CAD build for the part. Positions are in the model's coordinates, mm. A direction names the side the tool comes from. Give positions to 0.01 mm unless a question says otherwise; leave off trailing zeros. Order: outer loops, then holes, each group sorted by start corner. A loop starts at its lowest first (then second) coordinate and runs counter-clockwise, first axis right, second up. Notation, with made-up numbers: (25.5, 42) -> (83.5, 42) arc R23 cw to (83.5, 57) -> close; hole circle Ø11 at (3, 54.5). An arc over 180 degrees is marked (long way). Answer as CSV lines item,"result".
Autodesk Inventor part; units mm, degrees
sketch "Skizze1" plane through (0, 0, 0) normal (0, 1, 0) x (-1, 0, 0)
  line L0 (75, 67.5) -> (-75, 67.5)
  line L1 (-75, 67.5) -> (-75, -67.5)
  line L2 (-75, -67.5) -> (75, -67.5)
  line L3 (75, -67.5) -> (75, 67.5)
  line L4 (75, 67.5) -> (-75, -67.5) construction
  line L5 (-75, 67.5) -> (75, -67.5) construction
  point P0 (0, 0)
  dimension "d0" = 150
  dimension "d1" = 135
extrude "Extrusion1" add sketch "Skizze1" along normal mid plane 3
sketch "Skizze2" plane through (0, 1.5, 0) normal (0, 1, 0) x (1, 0, 0)
  line L0 (-75, 67.5) -> (-75, -67.5)
  line L1 (75, -67.5) -> (75, 67.5)
  line L2 (-75, -67.5) -> (75, -67.5)
  line L3 (75, -67.5) -> (75, -66)
  line L4 (75, -66) -> (-75, -66)
  line L5 (-75, -66) -> (-75, -67.5)
  point P0 (0, 0)
  dimension "d4" = 135
  dimension "d5" = 1.5
extrude "Extrusion2" add sketch "Skizze2" along normal blind 15
sketch "Skizze3" plane through (0, 0, 0) normal (1, 0, 0) x (0, 1, 0)
  line L0 (1.5, -67.5) -> (1.5, 66)
  line L1 (1.5, -67.5) -> (-1.5, -67.5)
  line L2 (-1.5, -67.5) -> (-1.5, -77.5)
  line L3 (-1.5, -77.5) -> (1.5, -77.5)
  line L4 (1.5, -77.5) -> (1.5, -67.5)
  line L5 (2, -78.5) -> (11.5, -78.5)
  line L6 (1.5, -77.5) -> (1.5, -78)
  line L7 (-1.5, -77.5) -> (-1.5, -79.5)
  arc A0 (1.5, -78) -> (2, -78.5) centre (2, -78) ccw
  line L8 (12, -78.5) -> (12, -80)
  line L9 (12, -80) -> (-1, -80)
  arc A1 (-1.5, -79.5) -> (-1, -80) centre (-1, -79.5) ccw
  line L10 (12, -78) -> (12, -78)
  arc A2 (11.5, -78.5) -> (12, -78) centre (11.5, -78) ccw
  line L11 (12, -78.5) -> (12, -78)
  point P0 (0, 0)
  dimension "d8" = 10
  dimension "d16" = 1.5
  dimension "d17" = 0.5
  dimension "d19" = 10
  dimension "d20" = 0.5
extrude "Extrusion3" add sketch "Skizze3" along normal mid plane 150
sketch "Skizze5" plane through (0, 0, 0) normal (0, 0, 1) x (1, 0, 0)
  line L0 (75, 16.5) -> (75, -1.5)
  line L1 (75, -1.5) -> (87, -1.5)
  line L2 (87.5, -1) -> (87.5, 12)
  line L3 (85.5, 12) -> (85.5, 12)
  line L4 (86, 11.5) -> (86, 2)
  arc A0 (86, 11.5) -> (85.5, 12) centre (85.5, 11.5) ccw
  line L5 (85.5, 12) -> (87.5, 12)
  line L6 (75, 1.5) -> (85.5, 1.5)
  line L7 (75, -1.5) -> (-75, -1.5)
  line L8 (75, -1.5) -> (75, 1.5)
  arc A1 (85.5, 1.5) -> (86, 2) centre (85.5, 2) ccw
  arc A2 (87, -1.5) -> (87.5, -1) centre (87, -1) ccw
  line L9 (-75, -1.5) -> (-75, 16.5)
  line L10 (-75, -1.5) -> (-87, -1.5)
  line L11 (-87.5, -1) -> (-87.5, 12)
  line L12 (-85.5, 12) -> (-85.5, 12)
  line L13 (-86, 11.5) -> (-86, 2)
  line L14 (-85.5, 1.5) -> (-75, 1.5)
  line L15 (-75, 1.5) -> (-75, -1.5)
  arc A3 (-85.5, 12) -> (-86, 11.5) centre (-85.5, 11.5) ccw
  line L16 (-87.5, 12) -> (-85.5, 12)
  arc A4 (-86, 2) -> (-85.5, 1.5) centre (-85.5, 2) ccw
  arc A5 (-87.5, -1) -> (-87, -1.5) centre (-87, -1) ccw
  point P0 (0, 0)
  point P1 (87.5, -1.5)
  point P2 (-87.5, -1.5)
  point P3 (-86, 12)
  point P4 (-86, 1.5)
  dimension "d39" = 13.5
  dimension "d42" = 0.5
  dimension "d43" = 0.5
  dimension "d44" = 12.5
  dimension "d45" = 1.5
  dimension "d46" = 2
  dimension "d48" = 10.5
  dimension "d49" = 12.5
  dimension "d50" = 13.5
  dimension "d51" = 2
  dimension "d52" = 10.5
  dimension "d53" = 0.5
  dimension "d54" = 0.5
extrude "Extrusion4" add sketch "Skizze5" along normal mid plane 135
properties part number "deckel"
1) Pin check, flat tips, straight feed: P1, Ø2, axis at x = 18, z = -79.5, coming from the +Y side; P2, Ø2, axis at x = -33, z = -33, coming from the +Y side; P3, Ø6, axis at x = 81, y = 6, coming from the -Z side. Stop position of each tip, or through.
Data:
P1,"stops at y = 12"
P2,"stops at y = 1.5"
P3,"passes through"
2) Which spindle directions (+Z, -Z, +X, -X, +Y, -Y) get a long thin tool onto all of the face, cutting with end or side? Do faces 4 (the flat face through (75, 1, -75)), 5 (the flat face through (-75, 1, -75)), 6 (the flat face through (86, 7, -1)), 7 (the flat face through (-1, 7, -78.5)), 8 (the flat face through (87.5, 5, -1)). Say none if no direction does.
Data:
face 4,"-Z, +X, +Y, -Y"
face 5,"-Z, -X, +Y, -Y"
face 6,"+Z, -Z"
face 7,"+X, -X"
face 8,"+Z, -Z, +X, +Y, -Y"
3) Band-saw the part on A-A, the plane y = 6.25. Write the cut outline in (x, z), then the cut area to 3 significant figures.
Data:
outline,"(-87.5, -67.5) -> (-86, -67.5) -> (-86, 67.5) -> (-87.5, 67.5) -> close; (-75, -80) -> (75, -80) -> (75, -78.5) -> (-75, -78.5) -> close; (-75, 66) -> (75, 66) -> (75, 67.5) -> (-75, 67.5) -> close; (86, -67.5) -> (87.5, -67.5) -> (87.5, 67.5) -> (86, 67.5) -> close"
area,"855 mm2"
4) Band-saw the part on B-B, the plane x = 11. Write the cut outline in (y, z).
Data:
outline,"(-1.5, -79.5) arc R0.5 ccw to (-1, -80) -> (12, -80) -> (12, -78) arc R0.5 cw to (11.5, -78.5) -> (2, -78.5) arc R0.5 cw to (1.5, -78) -> (1.5, 66) -> (16.5, 66) -> (16.5, 67.5) -> (-1.5, 67.5) -> close"
5) Pull direction Z, two halves, no side cores. Call faces 1 (the flat face through (-1, 6, -80)), 2 (the flat face through (1, 9, 66)), 3 (the flat face through (-87.5, 5, -1)): pulls with the +Z half, pulls with the -Z half, needs draft (parallel to the pull), parting line crosses it, or undercut.
Data:
face 1,"pulls with the -Z half"
face 2,"undercut"
face 3,"needs draft"
6) Band-saw the part on C-C, the plane z = -30. Write the cut outline in (x, y).
Data:
outline,"(-87.5, -1) arc R0.5 ccw to (-87, -1.5) -> (87, -1.5) arc R0.5 ccw to (87.5, -1) -> (87.5, 12) -> (85.5, 12) arc R0.5 cw to (86, 11.5) -> (86, 2) arc R0.5 cw to (85.5, 1.5) -> (-85.5, 1.5) arc R0.5 cw to (-86, 2) -> (-86, 11.5) arc R0.5 cw to (-85.5, 12) -> (-87.5, 12) -> close"
7) Wall check: line 1 along X through (y, z) = (8, 50.5); line 2 along Z through (x, y) = (-52, 4.75); line 3 along Z through (x, y) = (-18.5, 15). Give the ranges that are in metal, low to high. Write a range as [from, to].
Data:
line 1,"x = [-87.5, -86], [86, 87.5]"
line 2,"z = [-80, -78.5], [66, 67.5]"
line 3,"z = [66, 67.5]"
